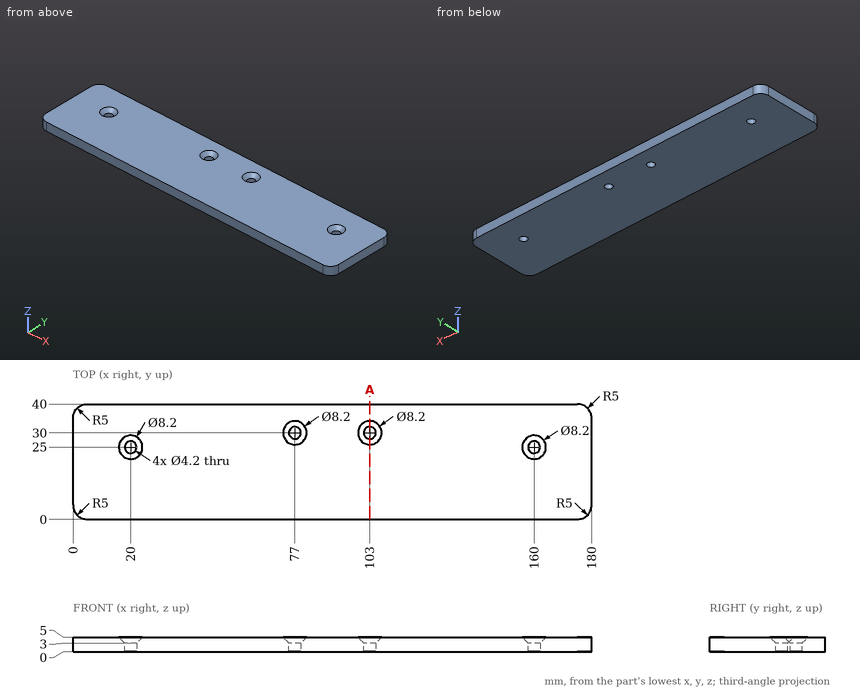
Part print with two shaded views. Sizes in mm from the minimum x, y, z corner. Coordinates: 2 decimals unless noted, no trailing zeros. Write each loop counter-clockwise with the first axis right and the second up, starting at its lowest first coordinate (ties: lowest second). Pieces come first, ordered by that corner, then holes. Notation, with made-up numbers: (36.25, 24.5) -> (75.25, 24.5) arc R25 ccw to (75.25, 38.5) -> close; hole circle Ø3 at (-38.5, 55). An arc over 180 degrees is marked (long way). Return JSON: item names as keys, results as strings. Group by question number.
Q1. Flat gauge pins, fed straight in: pin 1 (6.5 mm diameter, centred on x = 77, y = 30, fed in from +Z); pin 2 (1.5 mm diameter, centred on y = 12, z = 0.5, fed in from -X); pin 3 (5.5 mm diameter, centred on x = 160, y = 25, fed in from +Z). Where does each tip first touch, or does it go through?
Q2. Cut at A-A, the plane x = 103. Give the cut face in (y, z), then the cut area to 3 significant figures.
Q3. Drill centre lines: line 1 (Y direction, x = 77, z = 1.85); line 2 (X direction, y = 29.5, z = 0.65); line 3 (X direction, y = 31, z = 3.75). Where is each one in solid material? Low to high.
Returned:
{
 "1": {"pin 1": "stops at z = 4.15", "pin 2": "stops at x = 0", "pin 3": "stops at z = 3.65"},
 "2": {"outline": "(0, 0) -> (27.9, 0) -> (27.9, 3) -> (25.9, 5) -> (0, 5) -> close; (32.1, 0) -> (40, 0) -> (40, 5) -> (34.1, 5) -> (32.1, 3) -> close", "area": "175 mm2"},
 "3": {"line 1": "y = 0 to 27.9, 32.1 to 40", "line 2": "x = 0 to 74.96, 79.04 to 100.96, 105.04 to 180", "line 3": "x = 0 to 74.33, 79.67 to 100.33, 105.67 to 180"}
}
